from build123d import *

# Parameters (mm, degrees)
F0_W           = 45
F0_H           = 41
F0_R           = 6.25
F1_DEPTH       = 0.4
F5_D           = 13
F5_CSINK_D     = 20
F5_CSINK_ANGLE = 135
F7_W           = 2.3
F7_H           = 4


with BuildPart() as f1:
    # F0 (on Top) → F1 (new body)
    with BuildSketch(Plane.XY):
        Rectangle(F0_W, F0_H)
        with Locations((-11.75, -5)):
            Circle(F0_R, mode=Mode.SUBTRACT)
    extrude(amount=-F1_DEPTH)

    # F3 (on plane+point) → F4 (revolve)
    with BuildSketch(Plane.XZ.offset(-2)):
        Polygon((16.0175038762, 0), (6.2175038762, 0), (6.2175038762, -18), (14.4175038762, -18), align=None)
    revolve(axis=Axis((6.2175038762, 2, -9), (0, 0, -1)))

    # F5 (through all)
    with Locations(Plane.XY):
        with Locations((6.5, 2)):
            CounterSinkHole(F5_D / 2, F5_CSINK_D / 2, counter_sink_angle=F5_CSINK_ANGLE)

    # F7 (on plane+point) → F8 (revolve)
    with BuildSketch(Plane.XZ.offset(-15.55)):
        with Locations((13.9514571965, -2)):
            Rectangle(F7_W, F7_H)
    revolve(axis=Axis((12.8014571965, 15.55, -2), (0, 0, -1)))


solid = f1.part
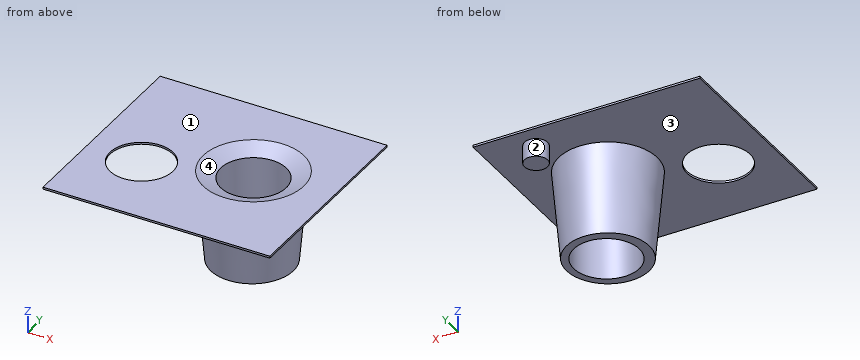
Here's how the part is built. I have some questions about the finished solid (model axes, mm). Face numbers are marked on the shaded views. A direction names the side the tool comes from. Give positions to 0.01 mm unless a question says otherwise; leave off trailing zeros. Order: outer loops, then holes, each group sorted by start corner. A loop starts at its lowest first (then second) coordinate and runs counter-clockwise, first axis right, second up. Notation, with made-up numbers: (64, 78.5) -> (90, 78.5) arc R31 cw to (90, 117.5) -> close; hole circle Ø6 at (-11.5, -23). An arc over 180 degrees is marked (long way). Use a Markdown table: item, result. Add a question column.
Item 1: Imagine slicing it at B-B on y = 2. Please give me the cut outline in (x, z), plus the area to 3 significant figures.
Item 2: Imagine slicing it at A-A on x = -11.75. Please give me the cut outline in (y, z), plus the area to 3 significant figures.
Item 3: For the marked faces 3 and 4, which set-ups out of +Z, -Z, +X, -X, +Y, -Y let a thin tool reach every point of the face, with its end or its side?
Item 4: Will these pins go through, and if not, where does the flat tip stop? pin 1 (10 mm diameter, centred on x = 11, y = -5, fed in from +Z); pin 2 (2 mm diameter, centred on y = 4, z = -9.5, fed in from +X); pin 3 (1.4 mm diameter, centred on x = 13.5, y = 14.5, fed in from -Z); pin 4 (8 mm diameter, centred on y = 3.5, z = -10, fed in from -X).
Item 5: I need wall thicknesses on line 1 (Y direction, x = -11.75, z = -0.2); line 2 (Z direction, x = 17.5, y = -11); line 3 (Y direction, x = 1, z = -8.5). Which ranges of each line are inside material? Lowest first, please.
Item 6: Imagine slicing it at C-C on y = 15.55. Please give me the cut outline in (x, z), plus the area to 3 significant figures.
Item 7: If we mould it in two halves opening along Y, with no side actions, what happens to the marked faces 1 and 2? For each: pulls with the +Y half, pulls with the -Y half, needs draft (parallel to the pull), parting line crosses it, or undercut.
Item 8: Imagine slicing it at D-D on z = -2.75. Please give me the cut outline in (x, y), plus the area to 3 significant figures.
Data:
| question | item | result |
|---|---|---|
| 1 | outline | (-22.5, -0.4) -> (-3.55, -0.4) -> (-1.98, -18) -> (0, -18) -> (0, -1.45) -> (-3.5, 0) -> (-22.5, 0) -> close; (13, -18) -> (14.42, -18) -> (15.98, -0.4) -> (22.5, -0.4) -> (22.5, 0) -> (16.5, 0) -> (13, -1.45) -> close |
| 1 | area | 95.1 mm² |
| 2 | outline | (-20.5, -0.4) -> (-11.25, -0.4) -> (-11.25, 0) -> (-20.5, 0) -> close; (1.25, -0.4) -> (20.5, -0.4) -> (20.5, 0) -> (1.25, 0) -> close |
| 2 | area | 11.4 mm² |
| 3 | face 3 | -Z |
| 3 | face 4 | +Z |
| 4 | pin 1 | stops at z = 0 |
| 4 | pin 2 | stops at x = 15.15 |
| 4 | pin 3 | stops at z = -4 |
| 4 | pin 4 | stops at x = -3.03 |
| 5 | line 1 | y = -20.5 to -11.25, 1.25 to 20.5 |
| 5 | line 2 | z = -0.4 to 0 |
| 5 | line 3 | y = -5.39 to -1.46, 5.46 to 9.39 |
| 6 | outline | (-22.5, -0.4) -> (10.5, -0.4) -> (10.5, -4) -> (15.1, -4) -> (15.1, -0.4) -> (22.5, -0.4) -> (22.5, 0) -> (-22.5, 0) -> close |
| 6 | area | 34.6 mm² |
| 7 | face 1 | needs draft |
| 7 | face 2 | undercut |
| 8 | outline | circle Ø19.11 at (6.22, 2); circle Ø4.6 at (12.8, 15.55); hole circle Ø13 at (6.5, 2) |
| 8 | area | 171 mm² |
